```python
from build123d import *

# Parameters (mm, degrees)
EXTRUDE_1_DEPTH     = 20
SKETCH_2_W          = 45.2
SKETCH_2_H          = 55.2
CUT_EXTRUDE_1_DEPTH = 12
SKETCH_4_W          = 40
SKETCH_4_H          = 25.9
SKETCH_4_H_2        = 4.2
CUT_EXTRUDE_2_DEPTH = 21
SKETCH_6_R          = 1.45
CUT_EXTRUDE_4_DEPTH = 9
SKETCH_8_R          = 1.45
CUT_EXTRUDE_6_DEPTH = 6
SKETCH_9_R          = 1.45
CUT_EXTRUDE_7_DEPTH = 6


with BuildPart() as part:
    # 草图1 → 凸台-拉伸1 (new body)
    with BuildSketch(Plane.XY):
        with BuildLine():
            Line((-19.75, 29.75), (19.75, 29.75))
            ThreePointArc((19.75, 29.75), (23.285533906, 28.285533906), (24.75, 24.75))
            Line((24.75, 24.75), (24.75, -24.75))
            ThreePointArc((24.75, -24.75), (23.285533906, -28.285533906), (19.75, -29.75))
            Line((19.75, -29.75), (-19.75, -29.75))
            ThreePointArc((-19.75, -29.75), (-23.285533906, -28.285533906), (-24.75, -24.75))
            Line((-24.75, -24.75), (-24.75, 24.75))
            ThreePointArc((-24.75, 24.75), (-23.285533906, 28.285533906), (-19.75, 29.75))
        make_face()
    extrude(amount=EXTRUDE_1_DEPTH)

    # 草图2 → 切除-拉伸1 (cut)
    with BuildSketch(Plane(origin=(0, 0, 0), x_dir=(-1, 0, 0), z_dir=(0, 0, -1))):
        Rectangle(SKETCH_2_W, SKETCH_2_H)
    extrude(amount=-CUT_EXTRUDE_1_DEPTH, mode=Mode.SUBTRACT)

    # 草图4 → 切除-拉伸2 (cut, through all)
    with BuildSketch(Plane.XY.offset(20)):
        with Locations((-0.75, 13.2)):
            Rectangle(SKETCH_4_W, SKETCH_4_H)
        with Locations((-0.75, -23.065049662)):
            Rectangle(SKETCH_4_W, SKETCH_4_H_2)
    extrude(amount=-CUT_EXTRUDE_2_DEPTH, mode=Mode.SUBTRACT)

    # 草图6 → 切除-拉伸4 (cut, through all)
    with BuildSketch(Plane(origin=(0, 0, 12), x_dir=(-1, 0, 0), z_dir=(0, 0, -1))):
        with Locations((16.862, -3.116)):
            Circle(SKETCH_6_R)
        with Locations((-15.138, -3.116)):
            Circle(SKETCH_6_R)
    extrude(amount=-CUT_EXTRUDE_4_DEPTH, mode=Mode.SUBTRACT)

    # 草图8 → 切除-拉伸6 (cut)
    with BuildSketch(Plane(origin=(0, 29.75, 0), x_dir=(1, 0, 0), z_dir=(0, 1, 0))):
        with Locations((-17.75, -10)):
            Circle(SKETCH_8_R)
        with Locations((18.25, -10)):
            Circle(SKETCH_8_R)
    extrude(amount=-CUT_EXTRUDE_6_DEPTH, mode=Mode.SUBTRACT)

    # 草图9 → 切除-拉伸7 (cut)
    with BuildSketch(Plane.XZ.offset(29.75)):
        with Locations((-10, 10)):
            Circle(SKETCH_9_R)
        with Locations((10, 10)):
            Circle(SKETCH_9_R)
    extrude(amount=-CUT_EXTRUDE_7_DEPTH, mode=Mode.SUBTRACT)


solid = part.part
```
Model file for the job. Use its own axes, mm. A direction names the side the tool comes from. Give positions to 0.01 mm unless a question says otherwise; leave off trailing zeros. Loops run counter-clockwise (first coordinate to the right, second up) from the corner with the lowest first, then second, coordinate; pieces in that order, holes last. Notation, with made-up numbers: (-22, 43) -> (-12, 43) arc R27 ccw to (-12, 74) -> close; hole circle Ø8 at (52, 47.5). An arc over 180 degrees is marked (long way). Write each question's results on one line, items separated by ' | '.
(1) Cut at B-B on z = 7.75. List the corners of the cut face in (x, y), and give its area (3 significant figures).
Geometry results:
outline: (-24.75, -24.75) arc R5 ccw to (-19.75, -29.75) -> (19.75, -29.75) arc R5 ccw to (24.75, -24.75) -> (24.75, 24.75) arc R5 ccw to (19.75, 29.75) -> (-19.75, 29.75) arc R5 ccw to (-24.75, 24.75) -> close; hole (-22.6, -27.6) -> (22.6, -27.6) -> (22.6, 27.6) -> (-22.6, 27.6) -> close | area: 429 mm²
(2) Tool access for faces 1 (the cylindrical face through (-11.15, -28.69, 9.12)), 2 (the cylindrical face through (-16.411, 28.69, 10.555)), 3 (the flat face through (5, -6, 12)), 4 (the flat face through (-1, -20.965, 16)), 5 (the cylindrical face through (-23.25, -28.32, 9.86)): list every direction of +Z, -Z, +X, -X, +Y, -Y with a clear straight run to the whole face (end or side of a thin tool).
Geometry results:
face 1: -Y | face 2: +Y | face 3: -Z | face 4: +Z, -Z | face 5: +Z, -Z, -X, -Y
(3) Cut at C-C on x = 18.25. List the corners of the cut face in (y, z), and give its area (3 significant figures).
Geometry results:
outline: (-29.75, 0) -> (-27.6, 0) -> (-27.6, 12) -> (-25.17, 12) -> (-25.17, 20) -> (-29.75, 20) -> close; (-20.97, 12) -> (0.25, 12) -> (0.25, 20) -> (-20.97, 20) -> close; (26.15, 12) -> (27.6, 12) -> (27.6, 11.45) -> (29.75, 11.45) -> (29.75, 20) -> (26.15, 20) -> close; (27.6, 0) -> (29.75, 0) -> (29.75, 8.55) -> (27.6, 8.55) -> close | area: 281 mm²
(4) Flat gauge pins, fed straight in: pin 1 Ø12 at (x, y) = (9.5, 10) entering from +Z; pin 2 Ø12 at (x, y) = (14, 20.5) entering from -Z; pin 3 Ø1.7 at (x, z) = (18.25, 10) entering from +Y. Where does each tip first touch, or does it go through?
Geometry results:
pin 1: passes through | pin 2: stops at z = 12 | pin 3: stops at y = -27.6
(5) Pull direction X, two halves, no side cores. Call faces 6 (the flat face through (22.6, 0, 6)), 7 (the flat face through (24, 2, 0)), 8 (the flat face through (-24.75, 0, 10)), 9 (the cylindrical face through (23.25, 28.32, 9.86)): released by +X, released by -X, zero draft, split by the parting line, or undercut.
Geometry results:
face 6: undercut | face 7: zero draft | face 8: released by -X | face 9: released by +X
(6) Probe line 1 along Y through (x, z) = (3, 15.25); line 2 along Z through (x, y) = (-10, -29); line 3 along X through (y, z) = (7, 10.25). List the from-to ranges inside material, lowest first.
Geometry results:
line 1: y = -29.75 to -25.17, -20.97 to 0.25, 26.15 to 29.75 | line 2: z = 0 to 8.55, 11.45 to 20 | line 3: x = -24.75 to -22.6, 22.6 to 24.75
(7) Cut at D-D on y = 2. List the corners of the cut face in (x, z).
Geometry results:
outline: (-24.75, 0) -> (-22.6, 0) -> (-22.6, 12) -> (-20.75, 12) -> (-20.75, 20) -> (-24.75, 20) -> close; (19.25, 12) -> (22.6, 12) -> (22.6, 0) -> (24.75, 0) -> (24.75, 20) -> (19.25, 20) -> close
(8) Cut at A-A on x = 6. List the corners of the cut face in (y, z).
Geometry results:
outline: (-29.75, 0) -> (-27.6, 0) -> (-27.6, 12) -> (-25.17, 12) -> (-25.17, 20) -> (-29.75, 20) -> close; (-20.97, 12) -> (0.25, 12) -> (0.25, 20) -> (-20.97, 20) -> close; (26.15, 12) -> (27.6, 12) -> (27.6, 0) -> (29.75, 0) -> (29.75, 20) -> (26.15, 20) -> close
